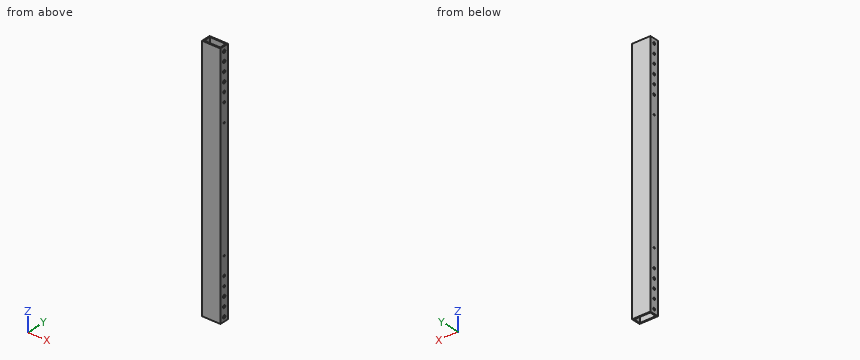
from build123d import *

# Parameters (mm, degrees)
BOSS_EXTRUDE1_DEPTH                   = 342.9
BOSS_EXTRUDE1_DEPTH_BACK              = 342.9
SKETCH3_W                             = 50.8
SKETCH3_H                             = 25.4
SKETCH3_W_2                           = 44.45
SKETCH3_H_2                           = 19.05
F_1_4_0_25_DIAMETER_HOLE4_AT_2_COUNT  = 2
F_1_4_0_25_DIAMETER_HOLE4_AT_2_PITCH  = 25.4
F_1_4_0_25_DIAMETER_HOLE5_D           = 6.35
F_1_4_0_25_DIAMETER_HOLE5_CSINK_D     = 7.9248
F_1_4_0_25_DIAMETER_HOLE5_CSINK_ANGLE = 82
F_1_4_0_25_DIAMETER_HOLE6_D           = 6.35
F_1_4_0_25_DIAMETER_HOLE7_D           = 6.35
F_1_4_0_25_DIAMETER_HOLE8_D           = 6.35
F_1_4_0_25_DIAMETER_HOLE8_CSINK_D     = 7.9248
F_1_4_0_25_DIAMETER_HOLE8_CSINK_ANGLE = 82
F_5_32_0_15625_DIAMETER_HOLE1_D       = 3.96875


with BuildPart() as part:
    # Sketch3 → Boss-Extrude1 (new, two sides: drawn at the far end of the back side and taken through both)
    with BuildSketch(Plane.XY.offset(-BOSS_EXTRUDE1_DEPTH_BACK)):
        Rectangle(SKETCH3_W, SKETCH3_H)
        Rectangle(SKETCH3_W_2, SKETCH3_H_2, mode=Mode.SUBTRACT)
    extrude(amount=BOSS_EXTRUDE1_DEPTH + BOSS_EXTRUDE1_DEPTH_BACK)

    # Sketch13 → 1/4 (0.25) Diameter Hole3 (revolve, cut)
    with BuildSketch(Plane(origin=(-25.4, 0, -330.911799988), x_dir=(0, 0, 1), z_dir=(0, 1, 0))):
        Polygon((0, 0), (0, 50.8), (3.9624, 50.8), (3.175, 49.894199916), (3.175, 0), align=None)
    revolve(axis=Axis((-31.75, 0, -330.911799988), (1, 0, 0)), mode=Mode.SUBTRACT)

    # Sketch15 → 1/4 (0.25) Diameter Hole4 (revolve, cut)
    with BuildSketch(Plane(origin=(-25.4, 0, 304.8), x_dir=(0, 0, 1), z_dir=(0, 1, 0))):
        Polygon((0, 0), (0, 50.8), (3.9624, 50.8), (3.175, 49.894199916), (3.175, 0), align=None)
    f_1_4_0_25_diameter_hole4 = revolve(axis=Axis((-31.75, 0, 304.8), (1, 0, 0)), mode=Mode.SUBTRACT)

    # 1/4 (0.25) Diameter Hole4 at 2: 1/4 (0.25) Diameter Hole4 ×2
    with Locations(*[(0, 0, i * F_1_4_0_25_DIAMETER_HOLE4_AT_2_PITCH) for i in range(1, F_1_4_0_25_DIAMETER_HOLE4_AT_2_COUNT)]):
        add(f_1_4_0_25_diameter_hole4, mode=Mode.SUBTRACT)

    # 1/4 (0.25) Diameter Hole5 (through all)
    with Locations(Plane(origin=(25.4, 0, 0), x_dir=(0, 0, -1), z_dir=(1, 0, 0))):
        with Locations((305.511799988, 0), (280.111799988, 0)):
            CounterSinkHole(F_1_4_0_25_DIAMETER_HOLE5_D / 2, F_1_4_0_25_DIAMETER_HOLE5_CSINK_D / 2, counter_sink_angle=F_1_4_0_25_DIAMETER_HOLE5_CSINK_ANGLE)

    # 1/4 (0.25) Diameter Hole6 (through all)
    with Locations(Plane(origin=(25.4, 0, 0), x_dir=(0, 0, -1), z_dir=(1, 0, 0))):
        with Locations((229.311799988, 0), (254.711799988, 0)):
            Hole(F_1_4_0_25_DIAMETER_HOLE6_D / 2)

    # 1/4 (0.25) Diameter Hole7 (through all)
    with Locations(Plane(origin=(25.4, 0, 0), x_dir=(0, 0, -1), z_dir=(1, 0, 0))):
        with Locations((-203.2, 0), (-228.6, 0)):
            Hole(F_1_4_0_25_DIAMETER_HOLE7_D / 2)

    # 1/4 (0.25) Diameter Hole8 (through all)
    with Locations(Plane(origin=(25.4, 0, 0), x_dir=(0, 0, -1), z_dir=(1, 0, 0))):
        with Locations((-279.4, 0), (-254, 0)):
            CounterSinkHole(F_1_4_0_25_DIAMETER_HOLE8_D / 2, F_1_4_0_25_DIAMETER_HOLE8_CSINK_D / 2, counter_sink_angle=F_1_4_0_25_DIAMETER_HOLE8_CSINK_ANGLE)

    # 5/32 (0.15625) Diameter Hole1 (through all)
    with Locations(Plane(origin=(25.4, 0, 0), x_dir=(0, 0, -1), z_dir=(1, 0, 0))):
        with Locations((-152.4, 0), (178.511799988, 0)):
            Hole(F_5_32_0_15625_DIAMETER_HOLE1_D / 2)


solid = part.part
Source: CAD feature listing. Evaluate the final solid. Frame: model axes, mm. Coordinates: 2 decimals unless noted, no trailing zeros. Loops run counter-clockwise (first coordinate to the right, second up) from the corner with the lowest first, then second, coordinate; pieces in that order, holes last. Notation, with made-up numbers: (35.5, 88) -> (67.5, 88) arc R18 ccw to (67.5, 102) -> close; hole circle Ø9 at (34.5, 45). An arc over 180 degrees is marked (long way). Answer in a Markdown table with one row per item. Add a question column.
Q1. Ray query, line 1 along Y through (x, z) = (21.5, 141) (3 decimals); line 2 along X through (y, z) = (-7.5, -177) (3 decimals); line 3 along Y through (x, z) = (-23, 228). Return the intervals inside material, ascending.
Q2. Section A-A on x = -10. Return the cut outline in (y, z) (3 decimals), and give its area (3 significant figures).
Q3. Contact query for flat-ended pins moving along their axis: pin 1 Ø5 at (y, z) = (0, -305.51) entering from -X; pin 2 Ø7.5 at (y, z) = (0, -280.11) entering from +X. Output: stop coordinate, or through.
Q4. Section B-B on z = 70. Return the cut outline in (x, y) (3 decimals), and give its area (3 significant figures).
Computed values:
| question | item | result |
|---|---|---|
| 1 | line 1 | y = -12.7 to -9.525, 9.525 to 12.7 |
| 1 | line 2 | x = -25.4 to -22.225, 22.225 to 25.4 |
| 1 | line 3 | y = -12.7 to -3.12, 3.12 to 12.7 |
| 2 | outline | (-12.7, -342.9) -> (-9.525, -342.9) -> (-9.525, 342.9) -> (-12.7, 342.9) -> close; (9.525, -342.9) -> (12.7, -342.9) -> (12.7, 342.9) -> (9.525, 342.9) -> close |
| 2 | area | 4,350 mm^2 |
| 3 | pin 1 | passes through |
| 3 | pin 2 | stops at x = 25.16 |
| 4 | outline | (-25.4, -12.7) -> (25.4, -12.7) -> (25.4, 12.7) -> (-25.4, 12.7) -> close; hole (-22.225, -9.525) -> (22.225, -9.525) -> (22.225, 9.525) -> (-22.225, 9.525) -> close |
| 4 | area | 444 mm^2 |
